Here's the drawing with two shaded views (mm, measured from the low corner). I have some questions. Give positions to 0.01 mm unless a question says otherwise; leave off trailing zeros. Write each loop counter-clockwise with the first axis right and the second up, starting at its lowest first coordinate (ties: lowest second). Pieces come first, ordered by that corner, then holes.
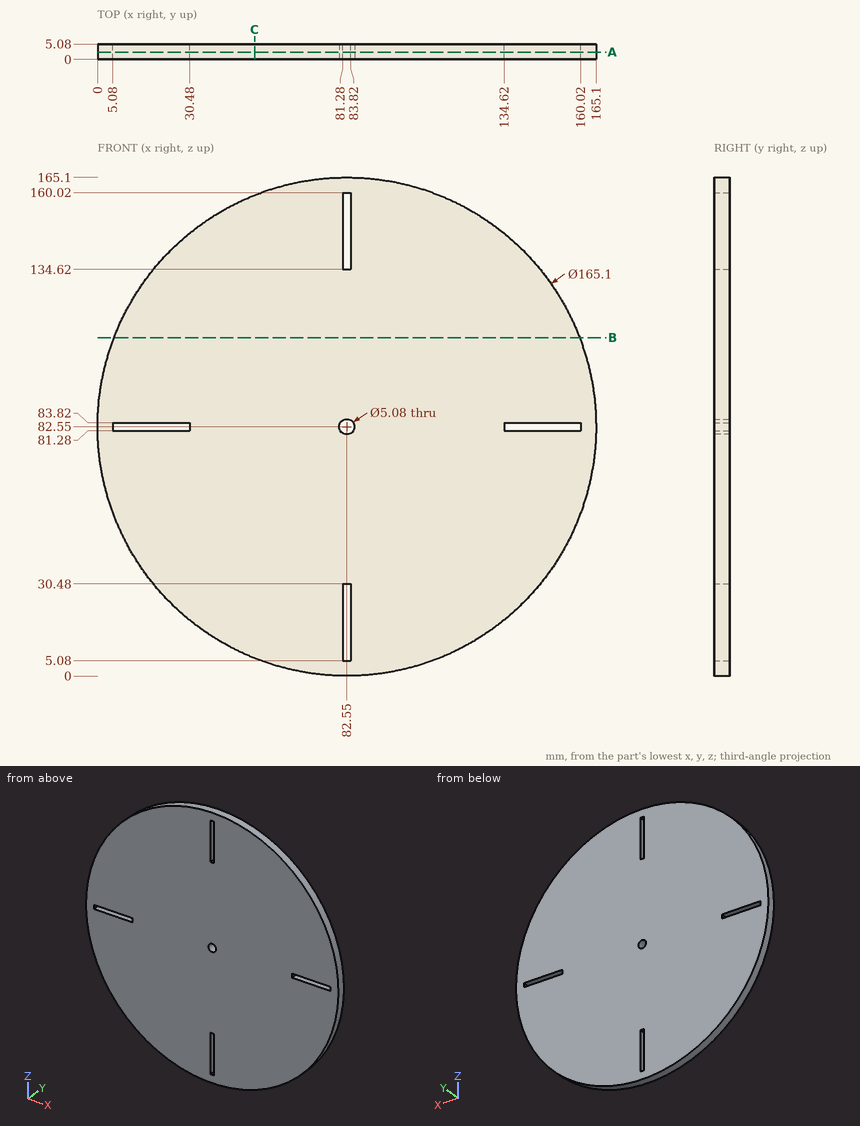
(1) If I drill on L1, parallel to X at y = 1.85, z = 82.55; L2, parallel to Z at x = 156.5, y = 2.3; L3, parallel to Z at x = 143, y = 0.8, over which ranges is the centre line in solid material (lowest first)?
Returned:
L1: x = 0 to 5.08, 30.48 to 80.01, 85.09 to 134.62, 160.02 to 165.1
L2: z = 45.86 to 81.28, 83.82 to 119.24
L3: z = 26.33 to 81.28, 83.82 to 138.77
(2) Will these pins go through, and if not, where does the flat tip stop? P1, Ø3, axis at x = 51, y = 2, coming from the -Z side; P2, Ø1.5, axis at y = 3, z = 142, coming from the -X side; P3, Ø1.5, axis at x = 147.5, y = 3.5, coming from the -Z side.
Returned:
P1: stops at z = 5.66
P2: stops at x = 24.51
P3: stops at z = 30.66
(3) Imagine slicing it at B-B, the plane z = 112. Write out the boundary of the cut face in (x, y).
Returned:
outline: (5.43, 0) - (159.67, 0) - (159.67, 5.08) - (5.43, 5.08) - close
(4) Imagine slicing it at C-C, the plane x = 52. Write out the boundary of the cut face in (y, z).
Returned:
outline: (0, 5.86) - (5.08, 5.86) - (5.08, 159.24) - (0, 159.24) - close
(5) Imagine slicing it at A-A, the plane y = 2.4. Write out the boundary of the cut face in (x, z).
Returned:
outline: circle Ø165.1 at (82.55, 82.55); hole (5.08, 81.28) - (30.48, 81.28) - (30.48, 83.82) - (5.08, 83.82) - close; hole circle Ø5.08 at (82.55, 82.55); hole (81.28, 5.08) - (83.82, 5.08) - (83.82, 30.48) - (81.28, 30.48) - close; hole (81.28, 134.62) - (83.82, 134.62) - (83.82, 160.02) - (81.28, 160.02) - close; hole (134.62, 81.28) - (160.02, 81.28) - (160.02, 83.82) - (134.62, 83.82) - close
